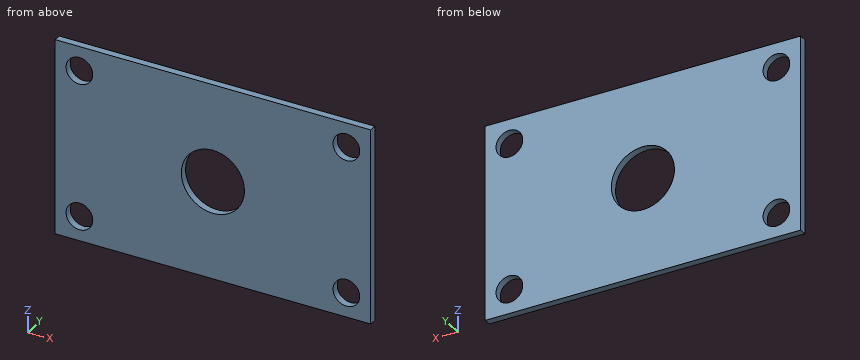
```python
from build123d import *

# Parameters (mm, degrees)
CROQUIS1_W              = 130
CROQUIS1_H              = 80
SALIENTE_EXTRUIR1_DEPTH = 3
CROQUIS2_R              = 13
CORTAR_EXTRUIR1_DEPTH   = 3
CROQUIS3_R              = 5.5
CORTAR_EXTRUIR2_DEPTH   = 3


with BuildPart() as part:
    # Croquis1 → Saliente-Extruir1 (new body)
    with BuildSketch(Plane(origin=(0, 0, 0), x_dir=(1, 0, 0), z_dir=(0, 1, 0))):
        Rectangle(CROQUIS1_W, CROQUIS1_H)
    extrude(amount=SALIENTE_EXTRUIR1_DEPTH)

    # Croquis2 → Cortar-Extruir1 (cut)
    with BuildSketch(Plane(origin=(0, 3, 0), x_dir=(1, 0, 0), z_dir=(0, 1, 0))):
        with Locations(Location((0, 0, 0), (0, 0, 270))):
            Circle(CROQUIS2_R)
    extrude(amount=-CORTAR_EXTRUIR1_DEPTH, mode=Mode.SUBTRACT)

    # Croquis3 → Cortar-Extruir2 (cut)
    with BuildSketch(Plane(origin=(0, 3, 0), x_dir=(1, 0, 0), z_dir=(0, 1, 0))):
        with Locations(Location((-55, 30, 0), (0, 0, 270))):
            Circle(CROQUIS3_R)
        with Locations(Location((-55, -30, 0), (0, 0, 270))):
            Circle(CROQUIS3_R)
        with Locations(Location((55, 30, 0), (0, 0, 270))):
            Circle(CROQUIS3_R)
        with Locations(Location((55, -30, 0), (0, 0, 270))):
            Circle(CROQUIS3_R)
    extrude(amount=-CORTAR_EXTRUIR2_DEPTH, mode=Mode.SUBTRACT)


solid = part.part
```
Geometry: final body of the model. Coordinates: model frame, mm. Round coordinates to 2 decimals unless told otherwise and drop trailing zeros. Order: outer loops, then holes, each group sorted by start corner. A loop starts at its lowest first (then second) coordinate and runs counter-clockwise, first axis right, second up. Notation, with made-up numbers: (61.25, -11) -> (96.25, -11) arc R18 cw to (96.25, 8) -> close; hole circle Ø2 at (16.25, 7.25). An arc over 180 degrees is marked (long way). Use one line per item in the form item = value.
(1) First-contact query: pin 1 Ø6.5 at (x, z) = (55, 30) entering from +Y; pin 2 Ø8 at (x, z) = (21, -7) entering from -Y. Flat tips, straight axial feed; report the tip coordinate or a pass-through.
Results list:
pin_1 = through
pin_2 = 0
(2) Section C-C on z = 30. Return loops of the section in (x, y).
Results list:
outline = (-65, 0) -> (-60.5, 0) -> (-60.5, 3) -> (-65, 3) -> close; (-49.5, 0) -> (49.5, 0) -> (49.5, 3) -> (-49.5, 3) -> close; (60.5, 0) -> (65, 0) -> (65, 3) -> (60.5, 3) -> close
(3) Ray query, probe 1 along X at (y, z) = (1.1, -30); probe 2 along Z at (x, y) = (-50.5, 2.85); probe 3 along X at (y, z) = (1.4, 27.5). Return the intervals inside material, ascending. Write a range as [from, to].
Results list:
probe_1 = [-65, -60.5], [-49.5, 49.5], [60.5, 65]
probe_2 = [-40, -33.16], [-26.84, 26.84], [33.16, 40]
probe_3 = [-65, -59.9], [-50.1, 50.1], [59.9, 65]
(4) Section B-B on x = -55. Return loops of the section in (y, z), and give its area (3 significant figures).
Results list:
outline = (0, -40) -> (3, -40) -> (3, -35.5) -> (0, -35.5) -> close; (0, -24.5) -> (3, -24.5) -> (3, 24.5) -> (0, 24.5) -> close; (0, 35.5) -> (3, 35.5) -> (3, 40) -> (0, 40) -> close
area = 174 mm^2
(5) Section D-D on x = 0. Return loops of the section in (y, z), and give its area (3 significant figures).
Results list:
outline = (0, -40) -> (3, -40) -> (3, -13) -> (0, -13) -> close; (0, 13) -> (3, 13) -> (3, 40) -> (0, 40) -> close
area = 162 mm^2
(6) Section A-A on z = 0. Return loops of the section in (x, y).
Results list:
outline = (-65, 0) -> (-13, 0) -> (-13, 3) -> (-65, 3) -> close; (13, 0) -> (65, 0) -> (65, 3) -> (13, 3) -> close
